Build history of the part. All positions in model axes, mm. Face numbers are marked on the shaded views. A direction names the side the tool comes from. Give positions to 0.01 mm unless a question says otherwise; leave off trailing zeros. Order: outer loops, then holes, each group sorted by start corner. A loop starts at its lowest first (then second) coordinate and runs counter-clockwise, first axis right, second up. Notation, with made-up numbers: (-28.5, -25.5) -> (-13.5, -25.5) arc R17 ccw to (-13.5, 7.5) -> close; hole circle Ø11 at (34, 2). An arc over 180 degrees is marked (long way). One line per item, written item: value. Start each with the question number.
(1) Pin check, flat tips, straight feed: pin 1 (5 mm diameter, centred on x = -3, z = -13.5, fed in from +Y); pin 2 (2 mm diameter, centred on x = -1, y = 2, fed in from +Z); pin 3 (1 mm diameter, centred on x = -1.5, y = -0.5, fed in from -Z). Stop position of each tip, or through.
(2) Saw through at C-C on z = -23. Give the cut face in (x, y), plus the area to 3 significant figures.
(3) Saw through at B-B on y = 0. Give the cut face in (x, z) (3 decimals).
(4) Saw through at D-D on z = -6. Give the cut face in (x, y) (3 decimals), plus the area to 3 significant figures.
(5) Probe line 1 (Z direction, x = -0.75, y = 0.25); line 2 (Z direction, x = 1.75, y = 0.25); line 3 (Y direction, x = 0.25, z = -3.5). List the from-to ranges inside material, lowest first.
(6) Which spindle directions (+Z, -Z, +X, -X, +Y, -Y) get a long thin tool onto all of the face, cutting with end or side? Do the marked faces 1 and 2. Say none if no direction does.
(7) Saw through at A-A on x = 0. Give the cut face in (y, z) (3 decimals), plus the area to 3 significant figures.
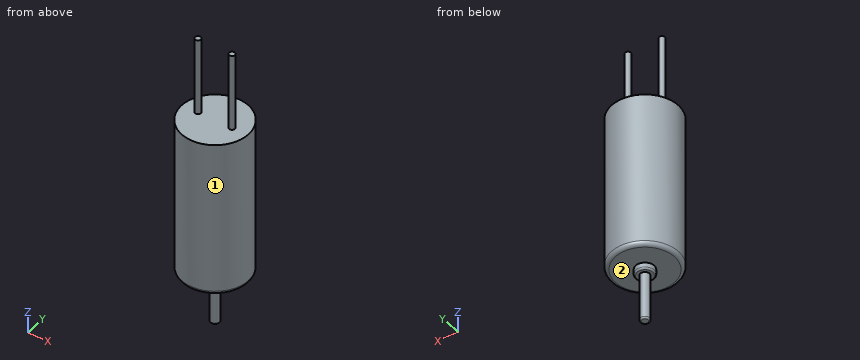
```python
from build123d import *

# Parameters (mm, degrees)
FILLET1_R           = 0.5
FILLET2_R           = 0.2
SKETCH2_R           = 0.375
BOSS_EXTRUDE1_DEPTH = 10


with BuildPart() as part:
    # Sketch1 → Revolve1 (revolve)
    with BuildSketch(Plane(origin=(0, 0, 0), x_dir=(1, 0, 0), z_dir=(0, 1, 0))):
        Polygon((4.325, 20.3), (4.325, 0), (0, 0), (0, 27.3), (0.6, 27.3), (0.6, 21.1), (1.2, 21.1), (1.2, 20.3), align=None)
    revolve(axis=Axis((0, 0, 0), (0, 0, -1)))

    # Fillet1
    fillet1_edges = [part.edges().sort_by_distance(p)[0] for p in [
        (-4.325, 0, -20.3),
    ]]
    fillet(fillet1_edges, radius=FILLET1_R)

    # Fillet2
    fillet2_edges = [part.edges().sort_by_distance(p)[0] for p in [
        (-1.2, 0, -21.1),
        (-0.6, 0, -27.3),
    ]]
    fillet(fillet2_edges, radius=FILLET2_R)

    # Sketch2 → Boss-Extrude1 (add)
    with BuildSketch(Plane.XY):
        with Locations((-2.25, 0)):
            Circle(SKETCH2_R)
        with Locations(Location((2.25, 0, 0), (0, 0, 180))):
            Circle(SKETCH2_R)
    extrude(amount=BOSS_EXTRUDE1_DEPTH)


solid = part.part
```
Results below:
1. pin 1: stops at y = 4.3
1. pin 2: stops at z = 0
1. pin 3: stops at z = -21.08
2. outline: circle Ø1.2 at (0, 0)
2. area: 1.13 mm²
3. outline: (-4.325, -19.8) arc R0.5 ccw to (-3.825, -20.3) -> (-1.2, -20.3) -> (-1.2, -20.9) arc R0.2 ccw to (-1, -21.1) -> (-0.6, -21.1) -> (-0.6, -27.1) arc R0.2 ccw to (-0.4, -27.3) -> (0.4, -27.3) arc R0.2 ccw to (0.6, -27.1) -> (0.6, -21.1) -> (1, -21.1) arc R0.2 ccw to (1.2, -20.9) -> (1.2, -20.3) -> (3.825, -20.3) arc R0.5 ccw to (4.325, -19.8) -> (4.325, 0) -> (2.625, 0) -> (2.625, 10) -> (1.875, 10) -> (1.875, 0) -> (-1.875, 0) -> (-1.875, 10) -> (-2.625, 10) -> (-2.625, 0) -> (-4.325, 0) -> close
4. outline: circle Ø8.65 at (0, 0)
4. area: 58.8 mm²
5. line 1: z = -21.1 to 0
5. line 2: z = -20.3 to 0
5. line 3: y = -4.32 to 4.32
6. face 1: +Z, -Z
6. face 2: -Z
7. outline: (-4.325, -19.8) arc R0.5 ccw to (-3.825, -20.3) -> (-1.2, -20.3) -> (-1.2, -20.9) arc R0.2 ccw to (-1, -21.1) -> (-0.6, -21.1) -> (-0.6, -27.1) arc R0.2 ccw to (-0.4, -27.3) -> (0.4, -27.3) arc R0.2 ccw to (0.6, -27.1) -> (0.6, -21.1) -> (1, -21.1) arc R0.2 ccw to (1.2, -20.9) -> (1.2, -20.3) -> (3.825, -20.3) arc R0.5 ccw to (4.325, -19.8) -> (4.325, 0) -> (-4.325, 0) -> close
7. area: 185 mm²
